Model file for the job. Use its own axes, mm. A direction names the side the tool comes from. Coordinates: 2 decimals unless noted, no trailing zeros. Write each loop counter-clockwise with the first axis right and the second up, starting at its lowest first coordinate (ties: lowest second). Pieces come first, ordered by that corner, then holes. Notation, with made-up numbers: M 78,7.5 L 123,7.5 A13 ccw 123,20.5 Z; hole C 63,41.5 d1. An arc over 180 degrees is marked long. One line per question, with ' | ' between items. Start each with the question number.
(1) Flat gauge pins, fed straight in: pin 1 Ø4 at (y, z) = (-38.5, -15.5) entering from -X; pin 2 Ø1.5 at (x, y) = (15.5, -10.5) entering from -Z; pin 3 Ø10 at (x, z) = (-11, 5.5) entering from -Y; pin 4 Ø8 at (x, y) = (-16, -37) entering from +Z. Where does each tip first touch, or does it go through?
(2) Tool access for faces 5 (the face through (-12.75, -22, 15)), 6 (the face through (13, -50, -3)), 7 (the face through (0, -37, -17.95)), 8 (the face through (12.75, -25, 0)), 9 (the face through (-32, 2, -12.75)): list every direction of +Z, -Z, +X, -X, +Y, -Y with a clear straight run to the whole face (end or side of a thin tool).
(3) Cut at D-D (x = -39). Write the cut outline in (y, z), plus the area to 4 significant figures.
(4) Cut at B-B (y = -36). Write the cut outline in (x, z), plus the area to 4 significant figures.
(5) Cut at C-C (z = 1.5). Write the cut outline in (x, y).
(6) Cut at A-A (x = 4.5). Write the cut outline in (y, z).
(7) Two-plate mould, pull along Z, no slides. Class faces 1 (the face through (-11, 0, -12)), 2 (the face through (-2, -37, -12.95)), 3 (the face through (0, -25, 12.75)), 4 (the face through (-31, 2, 12.75)): +Z half, -Z half, draft (parallel to the pull), parting line (faces both ways), or undercut.
(8) Wall check: probe 1 along Z at (x, y) = (11, -45); probe 2 along X at (y, z) = (-35, -6). Give the ranges that are in metal, low to high.
from build123d import *

# Parameters (mm, degrees)
BOSS_EXTRUDE1_DEPTH = 5
BOSS_EXTRUDE2_DEPTH = 5
SKETCH4_W           = 30.7
SKETCH4_H           = 55
BOSS_EXTRUDE3_DEPTH = 5
SKETCH5_W           = 35.5
SKETCH5_H           = 25
BOSS_EXTRUDE4_DEPTH = 5


with BuildPart() as part:
    # Sketch2 → Boss-Extrude1 (new body)
    with BuildSketch(Plane(origin=(0, 0, 0), x_dir=(1, 0, 0), z_dir=(0, 1, 0))):
        Polygon((-12.75, 12.75), (-12.75, 50), (12.75, 50), (12.75, -12.75), (-50, -12.75), (-50, 12.75), align=None)
    extrude(amount=BOSS_EXTRUDE1_DEPTH)

    # Sketch3 → Boss-Extrude2 (add)
    with BuildSketch(Plane.XY.offset(12.75)):
        Polygon((12.75, 0), (12.75, -50), (-12.75, -50), (-12.75, 0), (-12.75, 5), (12.75, 5), align=None)
    extrude(amount=BOSS_EXTRUDE2_DEPTH)

    # Sketch4 → Boss-Extrude3 (add)
    with BuildSketch(Plane(origin=(12.75, 0, 0), x_dir=(0, 0, -1), z_dir=(1, 0, 0))):
        with Locations((-2.4, -22.5)):
            Rectangle(SKETCH4_W, SKETCH4_H)
    extrude(amount=BOSS_EXTRUDE3_DEPTH)

    # Sketch5 → Boss-Extrude4 (add)
    with BuildSketch(Plane(origin=(0, 0, -12.95), x_dir=(-1, 0, 0), z_dir=(0, 0, -1))):
        with Locations((0, -37.5)):
            Rectangle(SKETCH5_W, SKETCH5_H)
    extrude(amount=BOSS_EXTRUDE4_DEPTH)


solid = part.part
Filled in:
1) pin 1: x = -17.75 | pin 2: z = -12.95 | pin 3: y = 0 | pin 4: z = 17.75
2) face 5: +Z, -X, +Y, -Y | face 6: +Z, -Z, +X, -X, -Y | face 7: -Z, +X, -X, -Y | face 8: -X, -Y | face 9: -Z, -X, +Y, -Y
3) outline: M 0,-12.75 L 5,-12.75 L 5,12.75 L 0,12.75 Z | area: 127.5 mm²
4) outline: M -17.75,-17.95 L 17.75,-17.95 L 17.75,17.75 L -12.75,17.75 L -12.75,12.75 L 12.75,12.75 L 12.75,-12.95 L -17.75,-12.95 Z | area: 458.5 mm²
5) outline: M -50,0 L 12.75,0 L 12.75,-50 L 17.75,-50 L 17.75,5 L -50,5 Z
6) outline: M -50,-17.95 L -25,-17.95 L -25,-12.95 L -50,-12.95 Z; M -50,12.75 L 0,12.75 L 0,-50 L 5,-50 L 5,17.75 L -50,17.75 Z
7) face 1: draft | face 2: undercut | face 3: undercut | face 4: +Z half
8) probe 1: -17.95 to -12.95, 12.75 to 17.75 | probe 2: 12.75 to 17.75
